```python
from build123d import *

# Parameters (mm, degrees)
F0_W     = 4
F0_H     = 14
F1_DEPTH = 25.4
F0_W_2   = 21.4
F0_R     = 1.6
F2_DEPTH = 4
F3_R     = 1.6
F4_DEPTH = 4
F5_F1_R  = 4
F5_F2_R  = 3.9999


# Not quite as in the source:
# - a fillet or chamfer is up to 0.001 mm smaller than in the source, because OpenCascade refuses the exact size


with BuildPart() as f1:
    # F0 (on Top) → F1 (new body)
    with BuildSketch(Plane.XY):
        with Locations((-8.6, 0)):
            Rectangle(F0_W, F0_H)
    extrude(amount=F1_DEPTH)

    # F0 (on Top) → F2 (join)
    with BuildSketch(Plane.XY):
        with Locations((4.1, 0)):
            Rectangle(F0_W_2, F0_H)
        Circle(F0_R, mode=Mode.SUBTRACT)
        with Locations((8.2, 0)):
            Circle(F0_R, mode=Mode.SUBTRACT)
    extrude(amount=F2_DEPTH)

    # F3 (on face) → F4 (cut, through all)
    with BuildSketch(Plane.YZ.offset(-6.6)):
        with Locations((0, 18.8)):
            Circle(F3_R)
        with Locations((0, 10.6)):
            Circle(F3_R)
    extrude(amount=-F4_DEPTH, mode=Mode.SUBTRACT)

    # F5: fillet of radius 4 on 5 edges, made by hand

    # F5_f1
    f5_f1_edges = [f1.edges().sort_by_distance(p)[0] for p in [
        (-6.6, 0, 4),
    ]]
    fillet(f5_f1_edges, radius=F5_F1_R)

    # F5_f2 (radius 4 in the source; OpenCascade refuses exactly that, so slightly less here)
    f5_f2_edges = [f1.edges().sort_by_distance(p)[0] for p in [
        (-6.6, 0, 25.4),
        (14.8, 0, 4),
        (-6.6, 7, 16.7),
        (6.1, -7, 4),
        (-5.4284271247, -7, 5.1715728753),
        (-5.4284271247, 7, 5.1715728753),
    ]]
    fillet(f5_f2_edges, radius=F5_F2_R)


solid = f1.part
```
Design review of the part built by this model. Coordinates are the model's own, in mm. A direction names the side the tool comes from. Coordinates: 2 decimals unless noted, no trailing zeros.
1) Add section B-B (y = 0). State how many separate pieces and enclosed holes the cut face has, plus the area to 3 significant figures.
2) Mouldability with a two-part tool opening along X and no side actions: class faces 1 (the flat face through (4, 0, 4)), 2 (the cylindrical face through (14.05, 0.1, 2.33)), 3 (the cylindrical face through (9.726, 0.481, 1.972)), 4 (the flat face through (-10.6, 0, 13)) as +X half, -X half, draft (parallel to the pull), parting line (faces both ways), or undercut.
3) Insertion check: pin 1 (6.5 mm diameter, centred on x = 2, y = 0.5, fed in from +Z); pin 2 (2 mm diameter, centred on x = 0.5, y = 5, fed in from +Z); pin 3 (4 mm diameter, centred on x = 9, y = -0.5, fed in from -Z); pin 4 (3 mm diameter, centred on x = -3, z = 3, fed in from -Y). Each pin has a flat end and moves straight along its axis. Give the tip position at first contact, or say it passes through.
4) To check wall thickness, follow L1, parallel to Z at x = -9, y = 0; L2, parallel to Y at x = 0, z = 1.4; L3, parallel to Z at x = -7.5, y = 0. State the ranges of each line that lie inside material, in increasing order.
5) Machinability: for faces 5 (the cylindrical face through (6.222, -5.859, 2.797)), 6 (the flat face through (-6.6, 0, 15)), 7 (the flat face through (2, 0, 0)), 8 (the cylindrical face through (5.978, 5.797, 2.859)), 9 (the flat face through (-9, -7, 1)), which of the approach directions +Z, -Z, +X, -X, +Y, -Y give a long, thin tool a straight path to every point of the face, cutting with its end or side? Answer none if there is none.
Check result:
1. separate pieces: 5
1. enclosed holes: 0
1. area: 133 mm2
2. face 1: draft
2. face 2: +X half
2. face 3: undercut
2. face 4: -X half
3. pin 1: stops at z = 4
3. pin 2: stops at z = 3.87
3. pin 3: stops at z = 0
3. pin 4: stops at y = -6.71
4. L1: z = 0 to 9, 12.2 to 17.2, 20.4 to 25.07
4. L2: y = -6.75 to -1.6, 1.6 to 6.75
4. L3: z = 0 to 9, 12.2 to 17.2, 20.4 to 23.93
5. face 5: +Z, +X, -Y
5. face 6: +Z, +X, +Y, -Y
5. face 7: -Z, +X, -X, +Y, -Y
5. face 8: +Z, +X, +Y
5. face 9: +Z, -Z, +X, -X, -Y
